```python
from build123d import *

# Parameters (mm, degrees)
ESQUISSE1_R                                   = 38
BOSS_EXTRU_1_DEPTH                            = 15
ESQUISSE4_R                                   = 35
ENL_V_MAT_EXTRU_1_DEPTH                       = 14.5
ESQUISSE9_R                                   = 38
BOSS_EXTRU_2_DEPTH                            = 20
BOSS_EXTRU_2_TAPER                            = 30
CONG_1_R                                      = 2
ESQUISSE7_W                                   = 6
ESQUISSE7_H                                   = 14.5
ENL_VEMENT_DE_MATI_RE_R_VOLUTION1_ANGLE       = 20
ENL_VEMENT_DE_MATI_RE_R_VOLUTION1_OTHER_ANGLE = 20
ENL_V_MAT_EXTRU_3_DEPTH                       = 65.132675714
ENL_V_MAT_EXTRU_3_DEPTH_BACK                  = 65.132675714
ESQUISSE10_W                                  = 90
ESQUISSE10_H                                  = 30
BOSS_EXTRU_3_REACH                            = 66.132
ESQUISSE14_W                                  = 3
ESQUISSE14_H                                  = 1.5
R_VOLUTION1_ANGLE                             = 4
ENL_V_MAT_EXTRU_4_DEPTH                       = 9


# Read off the part's stored shape, not the designer's step: Coque1
with BuildPart() as part:
    # Esquisse1 → Boss.-Extru.1 (new body)
    with BuildSketch(Plane(origin=(0, 0, 0), x_dir=(1, 0, 0), z_dir=(0, 1, 0))):
        with Locations(Location((0, 0, 0), (0, 0, 270))):
            Circle(ESQUISSE1_R)
    extrude(amount=BOSS_EXTRU_1_DEPTH)

    # Esquisse4 → Enlèv. mat.-Extru.1 (cut)
    with BuildSketch(Plane.XZ):
        with Locations(Location((0, 0, 0), (0, 0, 270))):
            Circle(ESQUISSE4_R)
    extrude(amount=-ENL_V_MAT_EXTRU_1_DEPTH, mode=Mode.SUBTRACT)

    # Esquisse9 → Boss.-Extru.2 (add)
    with BuildSketch(Plane(origin=(0, 15, 0), x_dir=(1, 0, 0), z_dir=(0, 1, 0))):
        with Locations(Location((0, 0, 0), (0, 0, 270))):
            Circle(ESQUISSE9_R)
    extrude(amount=BOSS_EXTRU_2_DEPTH, taper=BOSS_EXTRU_2_TAPER)

    # Congé1
    cong_1_edges = [part.edges().sort_by_distance(p)[0] for p in [
        (0, 35, -26.452994616),
        (0, 15, -38),
    ]]
    fillet(cong_1_edges, radius=CONG_1_R)

    # Esquisse7 → Enlèvement de matière-Révolution1 (revolve, cut)
    with BuildSketch(Plane(origin=(0, 0, 0), x_dir=(0, 0, -1), z_dir=(1, 0, 0))):
        with Locations((-35, 7.25)):
            Rectangle(ESQUISSE7_W, ESQUISSE7_H)
    revolve(axis=Axis((0, 0, 0), (0, 1, 0)), revolution_arc=ENL_VEMENT_DE_MATI_RE_R_VOLUTION1_ANGLE, mode=Mode.SUBTRACT)

    # Esquisse7 → Enlèvement de matière-Révolution1 other (revolve, cut)
    with BuildSketch(Plane(origin=(0, 0, 0), x_dir=(0, 0, -1), z_dir=(1, 0, 0))):
        with Locations((-35, 7.25)):
            Rectangle(ESQUISSE7_W, ESQUISSE7_H)
    revolve(axis=Axis((0, 0, 0), (0, -1, 0)), revolution_arc=ENL_VEMENT_DE_MATI_RE_R_VOLUTION1_OTHER_ANGLE, mode=Mode.SUBTRACT)

    # Coque1 outline → Coque1 (revolve, cut)
    with BuildSketch(Plane.XY):
        Polygon((34.824573519, 14.5), (24.720943809, 32), (0, 32), (0, 14.5), align=None)
    revolve(axis=Axis((0, 0, 0), (0, 1, 0)), mode=Mode.SUBTRACT)

    # Esquisse10 → Enlèv. mat.-Extru.3 (cut, two sides: drawn at the far end of the back side and taken through both)
    with BuildSketch(Plane(origin=(0, 0, 0), x_dir=(1, 0, 0), z_dir=(0, 1, 0)).offset(-ENL_V_MAT_EXTRU_3_DEPTH_BACK)):
        with Locations((0, 42)):
            Rectangle(ESQUISSE10_W, ESQUISSE10_H)
    extrude(amount=ENL_V_MAT_EXTRU_3_DEPTH + ENL_V_MAT_EXTRU_3_DEPTH_BACK, mode=Mode.SUBTRACT)

    # Esquisse13 → Boss.-Extru.3 (add, up to next)
    with BuildSketch(Plane(origin=(0, 0, 0), x_dir=(1, 0, 0), z_dir=(0, 1, 0)), mode=Mode.PRIVATE) as boss_extru_3_sk1:
        with BuildLine():
            Line((22.271057451, 27), (-22.271057451, 27))
            ThreePointArc((-22.271057451, 27), (-23.920345348, 25.55028529), (-25.475478406, 24))
            Line((-25.475478406, 24), (25.475478406, 24))
            ThreePointArc((25.475478406, 24), (23.920345348, 25.55028529), (22.271057451, 27))
        make_face()
    boss_extru_3_tool1 = extrude(boss_extru_3_sk1.sketch, amount=BOSS_EXTRU_3_REACH, mode=Mode.PRIVATE) - part.part
    add(boss_extru_3_tool1.solids().sort_by_distance((0, 0, -25.466594))[0])

    # Esquisse14 → Révolution1 (revolve)
    with BuildSketch(Plane(origin=(0, 0, 0), x_dir=(0, -1, 0), z_dir=(-0.500000000000001, 0, 0.866025403784438))):
        with Locations((-1.5, 34.25)):
            Rectangle(ESQUISSE14_W, ESQUISSE14_H)
        with Locations((-1.5, -34.25)):
            Rectangle(ESQUISSE14_W, ESQUISSE14_H)
    revolve(axis=Axis((0, 0, 0), (0, 1, 0)), revolution_arc=R_VOLUTION1_ANGLE)

    # Esquisse15 → Enlèv. mat.-Extru.4 (cut)
    with BuildSketch(Plane(origin=(0, 0, 0), x_dir=(1, 0, 0), z_dir=(0, 1, 0))):
        with BuildLine():
            Line((28.722813233, 20), (-28.722813233, 20))
            ThreePointArc((-28.722813233, 20), (0, 35), (28.722813233, 20))
        make_face()
    extrude(amount=ENL_V_MAT_EXTRU_4_DEPTH, mode=Mode.SUBTRACT)


solid = part.part
```
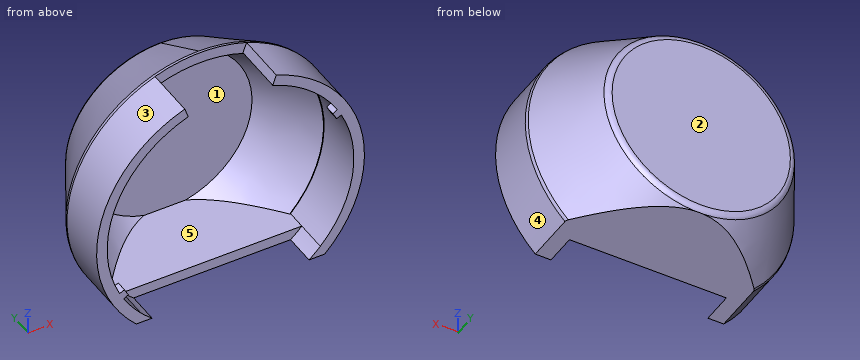
Geometry: final body of the model. Coordinates: model frame, mm. Face numbers are marked on the shaded views. A direction names the side the tool comes from. Give positions to 0.01 mm unless a question says otherwise; leave off trailing zeros. Loops run counter-clockwise (first coordinate to the right, second up) from the corner with the lowest first, then second, coordinate; pieces in that order, holes last. Notation, with made-up numbers: (86, -20) -> (102, -20) arc R12 ccw to (102, 1) -> close; hole circle Ø10 at (-6, 40). An arc over 180 degrees is marked (long way). Use CSV: the item, a comma, the result in double quotes.
(1) First-contact query: P1, Ø4, axis at y = 13, z = -8, coming from the -X side; P2, Ø5, axis at y = 11.5, z = -0.5, coming from the +X side; P3, Ø1.5, axis at x = -10, z = -25.5, coming from the -Y side; P4, Ø11.5, axis at x = 4.5, y = 17.5, coming from the +Z side. Flat tips, straight axial feed; report the tip coordinate or a pass-through.
From the geometry:
P1,"x = -37.52"
P2,"x = 38"
P3,"y = 9"
P4,"z = 38"
(2) Cut plane A-A (y = 4.5). Output: boundary loops of the cut face in (x, z), plus the area to 3 significant figures.
From the geometry:
outline,"(-26.74, -27) -> (-22.27, -27) arc R35 cw to (-11.97, 32.89) -> (-13, 35.71) arc R38 ccw to start; (11.97, 32.89) arc R35 cw to (22.27, -27) -> (26.74, -27) arc R38 ccw to (13, 35.71) -> close"
area,"450 mm^2"
(3) Access query for the marked faces 4 and 5. Directions: +Z, -Z, +X, -X, +Y, -Y. A direction counts if a zero-diameter tool reaches every point of the face in a straight line with its end or side. Return the directions, or none.
From the geometry:
face 4,"+X, +Y, -Y"
face 5,"-Y"
(4) Pull-direction query (Z, two-part tool) for the marked faces 1, 2 and 3; classes: released by +Z, released by -Z, zero draft, split by the parting line, or undercut.
From the geometry:
face 1,"undercut"
face 2,"zero draft"
face 3,"split by the parting line"
(5) Ray query, line 1 along Y through (x, z) = (-24, 3); line 2 along X through (y, z) = (15, 1.5); line 3 along Z through (x, y) = (-30.5, 4.5). Return the intervals inside material, ascending. Write a range as [from, to].
From the geometry:
line 1,"[32, 35]"
line 2,"[-37.9, -34.5], [34.5, 37.9]"
line 3,"[-22.67, -17.17], [17.17, 22.67]"
(6) Cut plane B-B (y = 24). Output: boundary loops of the cut face in (x, z), plus the area to 3 significant figures.
From the geometry:
outline,"(-18.63, -27) -> (18.63, -27) arc R32.8 ccw (long way) to start; hole (-16.88, -24) -> (16.88, -24) arc R29.34 ccw (long way) to start"
area,"652 mm^2"
